The listing builds one solid part. Answer for the finished solid, in the listing's coordinates (mm). A direction names the side the tool comes from. Round coordinates to 2 decimals unless told otherwise and drop trailing zeros. Write each loop counter-clockwise with the first axis right and the second up, starting at its lowest first coordinate (ties: lowest second). Pieces come first, ordered by that corner, then holes.
Item 1: Find section B-B on y = 59. Give the vertices of the cut face in (x, z) (3 decimals), then the cut area to 3 significant figures.
Item 2: Each of these flat-tipped pins is pushed along its axis until it touches: pin 1 (15 mm diameter, centred on y = 60, z = 14, fed in from +X); pin 2 (12 mm diameter, centred on x = 34.5, z = 12, fed in from +Y). Where does it stop, or does it pass through?
Item 3: Find section C-C on x = 7. Give the vertices of the cut face in (y, z), then the cut area to 3 significant figures.
Item 4: Find the intervals of material crossed by probe 1 along Y at (x, z) = (6.75, 15); probe 2 along Z at (x, y) = (5, 59); probe 3 along Y at (x, z) = (32.5, 8.75), in increasing order.
Item 5: Find section D-D on y = 7. Give the vertices of the cut face in (x, z), then the cut area to 3 significant figures.
Item 6: Find section A-A on x = 56.5. Give the vertices of the cut face in (y, z), then the cut area to 3 significant figures.
Item 7: For a pull along X with two mould halves and no side action, classify faces 4 (the face through (22, 7.6, 30)), 5 (the face through (30, 4, 11.5)), 6 (the face through (0, 41, 15)) as +X half, -X half, draft (parallel to the pull), parting line (faces both ways), or undercut.
Item 8: A tool of negligible diameter and unlimited length cuts with its end or side. For faces 1 (the face through (45, 8, 15)), 2 (the face through (80, 4, 15)), 3 (the face through (68.5, 4.1, 14.9)), from which of +Z, -Z, +X, -X, +Y, -Y can it reach the whole face along a straight path? Write none if from no direction.
```python
from build123d import *

# Parameters (mm, degrees)
EXTRUDE_1_DEPTH                     = 30
CUT_EXTRUDE_1_DEPTH                 = 60
HOLE_WIZARD_15_5_15_5_1_D           = 15.5
HOLE_WIZARD_15_5_15_5_1_DEPTH       = 17
HOLE_WIZARD_15_5_15_5_1_CSINK_D     = 15.55
HOLE_WIZARD_15_5_15_5_1_CSINK_ANGLE = 90
HOLE_WIZARD_15_5_15_5_1_TIP         = 4.656669797


with BuildPart() as part:
    # 草图1 → 凸台-拉伸1 (new body)
    with BuildSketch(Plane.XY):
        Polygon((0, 80), (0, 0), (80, 0), (80, 8), (8, 8), (8, 80), align=None)
    extrude(amount=EXTRUDE_1_DEPTH)

    # 草图2 → 切除-拉伸1 (cut)
    with BuildSketch(Plane(origin=(0, 8, 0), x_dir=(1, 0, 0), z_dir=(0, 1, 0))):
        with BuildLine():
            Line((55, -11.5), (65, -11.5))
            ThreePointArc((65, -11.5), (68.5, -15), (65, -18.5))
            Line((65, -18.5), (55, -18.5))
            ThreePointArc((55, -18.5), (51.5, -15), (55, -11.5))
        make_face()
        with BuildLine():
            Line((25, -11.5), (35, -11.5))
            ThreePointArc((35, -11.5), (38.5, -15), (35, -18.5))
            Line((35, -18.5), (25, -18.5))
            ThreePointArc((25, -18.5), (21.5, -15), (25, -11.5))
        make_face()
    extrude(amount=-CUT_EXTRUDE_1_DEPTH, mode=Mode.SUBTRACT)

    # Ø15.5 (15.5) 直径槽口1
    with Locations(Plane.ZY):
        with Locations((15, 59)):
            CounterSinkHole(HOLE_WIZARD_15_5_15_5_1_D / 2, HOLE_WIZARD_15_5_15_5_1_CSINK_D / 2, depth=HOLE_WIZARD_15_5_15_5_1_DEPTH, counter_sink_angle=HOLE_WIZARD_15_5_15_5_1_CSINK_ANGLE)
            with Locations((0, 0, -(HOLE_WIZARD_15_5_15_5_1_DEPTH + HOLE_WIZARD_15_5_15_5_1_TIP / 2))):  # 118° drill point
                Cone(0, HOLE_WIZARD_15_5_15_5_1_D / 2, HOLE_WIZARD_15_5_15_5_1_TIP, mode=Mode.SUBTRACT)


solid = part.part
```
Check values:
1. outline: (0, 0) - (8, 0) - (8, 7.25) - (0.025, 7.25) - (0, 7.225) - close; (0, 22.775) - (0.025, 22.75) - (8, 22.75) - (8, 30) - (0, 30) - close
1. area: 116 mm2
2. pin 1: stops at x = 8
2. pin 2: stops at y = 8
3. outline: (0, 0) - (80, 0) - (80, 30) - (0, 30) - close; hole circle Ø15.5 at (59, 15)
3. area: 2,210 mm2
4. probe 1: y = 0 to 51.25, 66.75 to 80
4. probe 2: z = 0 to 7.25, 22.75 to 30
4. probe 3: y = 0 to 8
5. outline: (0, 0) - (80, 0) - (80, 30) - (0, 30) - close; hole (25, 11.5) - (35, 11.5) arc R3.5 ccw to (35, 18.5) - (25, 18.5) arc R3.5 ccw to start; hole (55, 11.5) - (65, 11.5) arc R3.5 ccw to (65, 18.5) - (55, 18.5) arc R3.5 ccw to start
5. area: 2,180 mm2
6. outline: (0, 0) - (8, 0) - (8, 11.5) - (0, 11.5) - close; (0, 18.5) - (8, 18.5) - (8, 30) - (0, 30) - close
6. area: 184 mm2
7. face 4: draft
7. face 5: undercut
7. face 6: -X half
8. face 1: +Z, -Z, +X, +Y
8. face 2: +Z, -Z, +X, +Y, -Y
8. face 3: +Y, -Y
